The figure shows three views and two pictorial views of one solid part (mm, origin at its lowest corner). Answer the questions. A direction names the side the tool comes from. Give positions to 0.01 mm unless a question says otherwise; leave off trailing zeros. Write each loop counter-clockwise with the first axis right and the second up, starting at its lowest first coordinate (ties: lowest second). Pieces come first, ordered by that corner, then holes. Notation, with made-up numbers: (-20.75, 26) - (-2.75, 26) arc R26 cw to (-2.75, 53) - close; hole circle Ø6 at (-7.75, -12). An arc over 180 degrees is marked (long way). One line per question, with ' | ' between items. Start each with the question number.
1. A cutting plane is placed at A-A (x = 25). Determine the outline of the cut face in (y, z).
2. A cutting plane is placed at D-D (z = 9.5). Determine the outline of the cut face in (x, y), then the cut area to 3 significant figures.
3. A cutting plane is placed at B-B (z = 15). Determine the outline of the cut face in (x, y).
4. Given P1, Ø0.8, axis at y = 3.5, z = 18.5, coming from the -X side; P2, Ø2, axis at x = 20.5, z = 14.5, coming from the +Y side, each flat-ended and moving along its own axis, determine where each tip first touches the part or whether it passes through.
5. A cutting plane is placed at C-C (y = 0.95). Determine the outline of the cut face in (x, z), then the cut area to 3 significant figures.
6. For the marked faces 4 and 5, determine the directions among +Z, -Z, +X, -X, +Y, -Y from which every point of the face is accessible in a straight line to the end or side of a thin tool.
7. The mould has two halves that part along X. Classify the marked faces 1, 2 and 3: +X half, -X half, draft (parallel to the pull), parting line (faces both ways), or undercut.
8. Find the intervals of material crossed by L1, parallel to X at y = 1.45, z = 5; L2, parallel to X at y = 3.3, z = 9.5; L3, parallel to Z at x = 25, y = 1.5, in increasing order. Write a range as from..to.
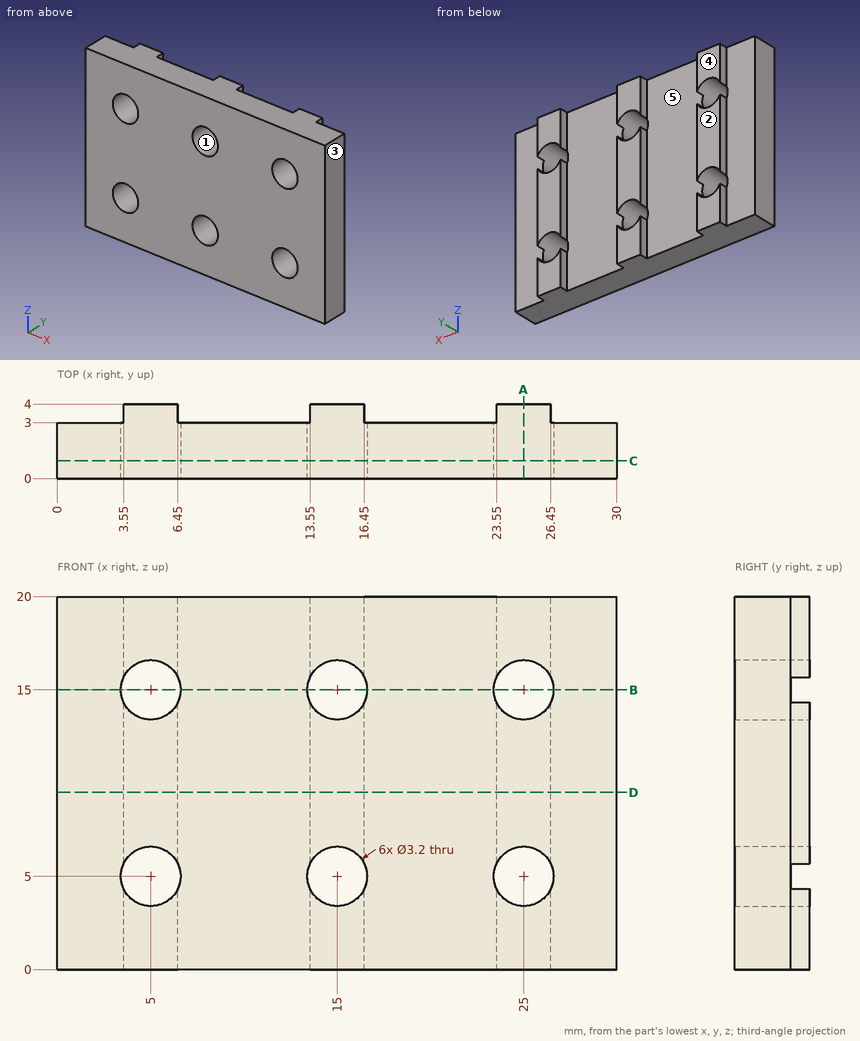
Determined:
1) outline: (0, 0) - (4, 0) - (4, 3.4) - (0, 3.4) - close; (0, 6.6) - (4, 6.6) - (4, 13.4) - (0, 13.4) - close; (0, 16.6) - (4, 16.6) - (4, 20) - (0, 20) - close
2) outline: (0, 0) - (30, 0) - (30, 3) - (26.45, 3) - (26.45, 4) - (23.55, 4) - (23.55, 3) - (16.45, 3) - (16.45, 4) - (13.55, 4) - (13.55, 3) - (6.45, 3) - (6.45, 4) - (3.55, 4) - (3.55, 3) - (0, 3) - close | area: 98.7 mm2
3) outline: (0, 0) - (3.4, 0) - (3.4, 3) - (0, 3) - close; (6.6, 0) - (13.4, 0) - (13.4, 3) - (6.6, 3) - close; (16.6, 0) - (23.4, 0) - (23.4, 3) - (16.6, 3) - close; (26.6, 0) - (30, 0) - (30, 3) - (26.6, 3) - close
4) P1: x = 3.55 | P2: y = 3
5) outline: (0, 0) - (30, 0) - (30, 20) - (0, 20) - close; hole circle Ø3.2 at (5, 5); hole circle Ø3.2 at (5, 15); hole circle Ø3.2 at (15, 5); hole circle Ø3.2 at (15, 15); hole circle Ø3.2 at (25, 5); hole circle Ø3.2 at (25, 15) | area: 552 mm2
6) face 4: +Z, -Z, +X, -X, +Y | face 5: +Z, -Z, +Y
7) face 1: undercut | face 2: draft | face 3: +X half
8) L1: 0..3.4, 6.6..13.4, 16.6..23.4, 26.6..30 | L2: 3.55..6.45, 13.55..16.45, 23.55..26.45 | L3: 0..3.4, 6.6..13.4, 16.6..20
